CAD build for the part. Positions are in the model's coordinates, mm. Coordinates: 2 decimals unless noted, no trailing zeros. Loops run counter-clockwise (first coordinate to the right, second up) from the corner with the lowest first, then second, coordinate; pieces in that order, holes last. Notation, with made-up numbers: (13.5, -36) -> (17.5, -36) arc R27 cw to (17.5, -19) -> close; hole circle Ø10 at (18.5, 83). An arc over 180 degrees is marked (long way). Write each question's results on one line, items separated by ' | '.
from build123d import *

# Parameters (mm, degrees)
F1_DEPTH = 0.635
F3_DEPTH = 25.4


with BuildPart() as f1:
    # F0 (on Front) → F1 (new body)
    with BuildSketch(Plane.XZ):
        with BuildLine():
            ThreePointArc((-0.8255, 0), (0, 0.8255), (0.8255, 0))
            Line((0.8255, 0), (1.905, 0))
            Line((1.905, 0), (0.9788597992, 9.1155531579))
            ThreePointArc((0.9788597992, 9.1155531579), (0.6596235144, 9.7461380267), (0, 10))
            ThreePointArc((0, 10), (-0.6596235144, 9.7461380267), (-0.9788597992, 9.1155531579))
            Line((-0.9788597992, 9.1155531579), (-1.905, 0))
            Line((-1.905, 0), (-0.8255, 0))
        make_face()
        with BuildLine():
            ThreePointArc((-0.8255, 0), (0, -0.8255), (0.8255, 0))
            Line((0.8255, 0), (-0.8255, 0))
        make_face()
        with BuildLine():
            Line((-0.8255, 0), (0.8255, 0))
            ThreePointArc((0.8255, 0), (0, 0.8255), (-0.8255, 0))
        make_face()
    extrude(amount=F1_DEPTH)

    # F2 (on face) → F3 (cut)
    with BuildSketch(Plane.XZ):
        with BuildLine():
            Line((-0.635, 0), (0.635, 0))
            ThreePointArc((0.635, 0), (0, 0.635), (-0.635, 0))
        make_face()
        with BuildLine():
            ThreePointArc((-0.635, 0), (0, -0.635), (0.635, 0))
            Line((0.635, 0), (-0.635, 0))
        make_face()
    extrude(amount=F3_DEPTH, mode=Mode.SUBTRACT)


solid = f1.part
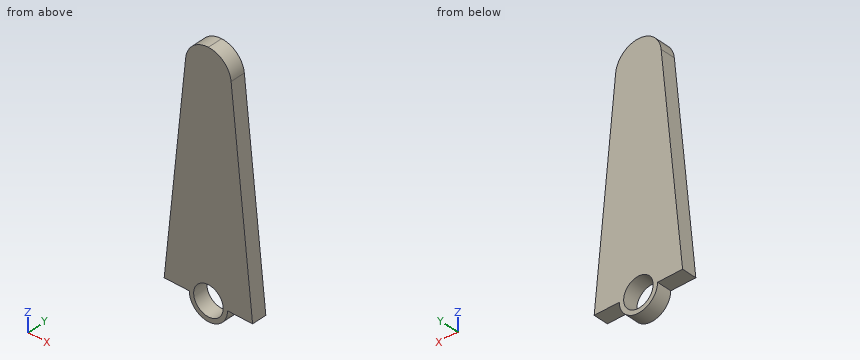
1) Slice it at A-A (y = -0.1). Write the cut outline in (x, z) (1 decimal), then the cut area to 3 significant figures.
Outcome:
outline: (-1.9, 0) -> (-0.8, 0) arc R0.8 ccw to (0.8, 0) -> (1.9, 0) -> (1, 9.1) arc R1 ccw to (-1, 9.1) -> close; hole circle Ø1.3 at (0, 0) | area: 27.4 mm^2
2) Slice it at D-D (z = 6). Write the cut outline in (x, y) (3 decimals), then the cut area to 3 significant figures.
Outcome:
outline: (-1.295, -0.635) -> (1.295, -0.635) -> (1.295, 0) -> (-1.295, 0) -> close | area: 1.65 mm^2
3) Slice it at C-C (x = 0.2). Write the cut outline in (y, z) (3 decimals).
Outcome:
outline: (-0.635, -0.801) -> (0, -0.801) -> (0, -0.603) -> (-0.635, -0.603) -> close; (-0.635, 0.603) -> (0, 0.603) -> (0, 9.979) -> (-0.635, 9.979) -> close
4) Drill centre lines: L1, parallel to Z at x = -0.45, y = -0.1; L2, parallel to X at y = -0.05, z = 8; L3, parallel to X at y = -0.5, z = 3. Where is each one in solid material? Low to high. Write a range as from..to.
Outcome:
L1: z = -0.69..-0.45, 0.45..9.89 | L2: x = -1.09..1.09 | L3: x = -1.6..1.6
5) Slice it at B-B (z = 0.5). Write the cut outline in (x, y) (3 decimals), then the cut area to 3 significant figures.
Outcome:
outline: (-1.854, -0.635) -> (-0.391, -0.635) -> (-0.391, 0) -> (-1.854, 0) -> close; (0.391, -0.635) -> (1.854, -0.635) -> (1.854, 0) -> (0.391, 0) -> close | area: 1.86 mm^2
